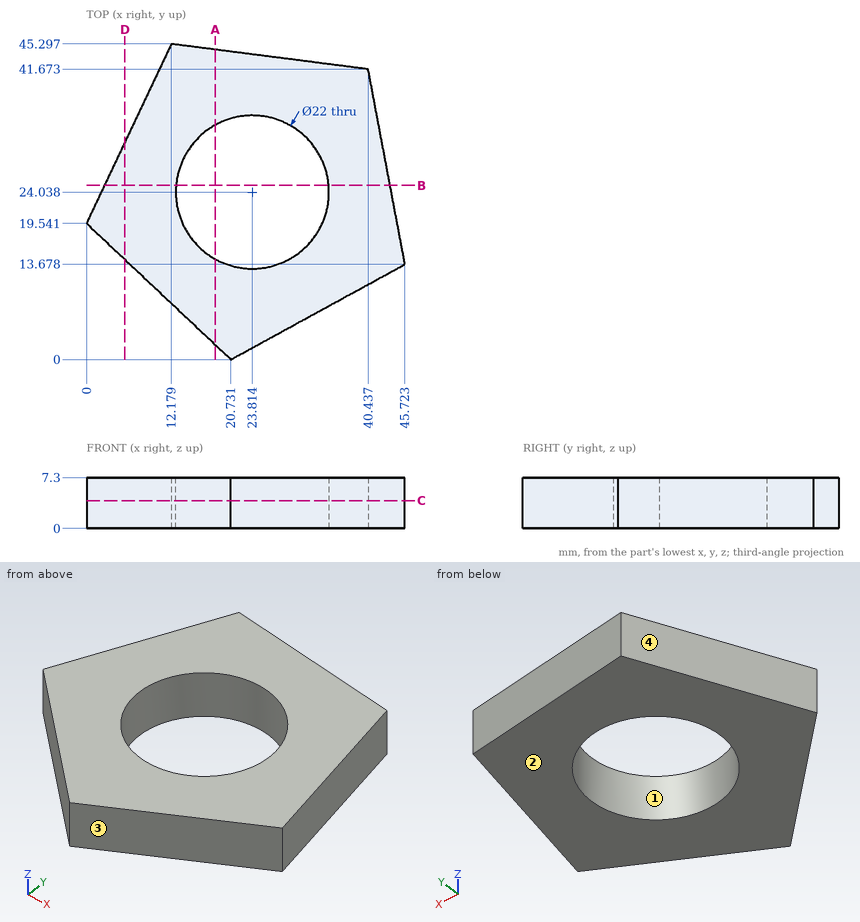
Study the drawing (mm; zero at the part's minimum x, y, z) and answer. Coordinates: 2 decimals unless noted, no trailing zeros. Write each loop counter-clockwise with the first axis right and the second up, starting at its lowest first coordinate (ties: lowest second). Pieces come first, ordered by that corner, then holes. Notation, with made-up numbers: (29.5, 13.25) - (40.5, 13.25) arc R21 cw to (40.5, 20.25) - close; hole circle Ø9 at (38.25, 35.25). An arc over 180 degrees is marked (long way). Put each result on its own line as item: value.
1. The part is cut by section C-C on z = 4. Give the vertices of the cut face in (x, y), plus the area to 3 significant figures.
Answer sheet:
outline: (0, 19.54) - (20.73, 0) - (45.72, 13.68) - (40.44, 41.67) - (12.18, 45.3) - close; hole circle Ø22 at (23.81, 24.04)
area: 1,020 mm^2
2. Determine the mould class of the marked faces 1, 2, 3 and 4 for opening direction Y: pulls with the +Y half, pulls with the -Y half, needs draft (parallel to the pull), parting line crosses it, or undercut.
Answer sheet:
face 1: undercut
face 2: needs draft
face 3: pulls with the -Y half
face 4: pulls with the +Y half
3. The part is cut by section B-B on y = 25. Give the vertices of the cut face in (x, z) (1 decimal), plus the area to 3 significant figures.
Answer sheet:
outline: (2.6, 0) - (12.9, 0) - (12.9, 7.3) - (2.6, 7.3) - close; (34.8, 0) - (43.6, 0) - (43.6, 7.3) - (34.8, 7.3) - close
area: 139 mm^2
4. Flat-ended cylindrical pins translate along their axes: pin 1 Ø3 at (x, z) = (10.5, 3) entering from +Y; pin 2 Ø2 at (y, z) = (16, 3.5) entering from -X (1 decimal); pin 3 Ø2 at (x, z) = (4.5, 1.5) entering from +Y (1 decimal). Find the tip coordinate at first contact, or state that the pin passes through.
Answer sheet:
pin 1: stops at y = 44.92
pin 2: stops at x = 2.7
pin 3: stops at y = 31.2
5. The part is cut by section A-A on x = 18.5. Give the vertices of the cut face in (y, z).
Answer sheet:
outline: (2.1, 0) - (14.41, 0) - (14.41, 7.3) - (2.1, 7.3) - close; (33.67, 0) - (44.49, 0) - (44.49, 7.3) - (33.67, 7.3) - close
6. The part is cut by section D-D on x = 5.5. Give the vertices of the cut face in (y, z).
Answer sheet:
outline: (14.36, 0) - (31.17, 0) - (31.17, 7.3) - (14.36, 7.3) - close
7. Find the intervals of material crossed by line 1 along X through (y, z) = (24.5, 4.75) (1 decimal); line 2 along Y through (x, z) = (32, 4) (1 decimal); line 3 along Y through (x, z) = (32.5, 6.25) (1 decimal), in increasing order. Write a range as from..to.
Answer sheet:
line 1: x = 2.3..12.8, 34.8..43.7
line 2: y = 6.2..16.7, 31.4..42.8
line 3: y = 6.4..17.3, 30.8..42.7
